Model file for the job. Use its own axes, mm. A direction names the side the tool comes from. Give positions to 0.01 mm unless a question says otherwise; leave off trailing zeros. Write each loop counter-clockwise with the first axis right and the second up, starting at its lowest first coordinate (ties: lowest second). Pieces come first, ordered by that corner, then holes. Notation, with made-up numbers: (60.5, -17.5) - (104.5, -17.5) arc R14 ccw to (104.5, -4.5) - close; hole circle Ø2 at (-20, 81.5). An arc over 180 degrees is marked (long way). One line per item, written item: value. Start each with the question number.
(1) Mould opens along Z. For faces 3 (the face through (-8.617, 13.461, 38.805)), 4 (the face through (-9.1, 28.575, -9.1)), 5 (the face through (-2.75, 22.31, 12.4)) say: pulls with the +Z half, pulls with the -Z half, needs draft (parallel to the pull), parting line crosses it, or undercut.
(2) Drop flat-ended pins along their axis: P1, Ø4.5, axis at x = 0, z = 51.63, coming from the +Y side; P2, Ø6, axis at x = 4.5, y = 20.5, coming from the -Z side; P3, Ø6, axis at x = -32.5, y = 9.5, coming from the +Z side. Give the stop position or say it passes through.
(3) Probe L1, parallel to Z at x = 0, y = -2; L2, parallel to X at y = 20.5, z = 0. List the from-to ranges inside material, lowest first.
(4) Cut at C-C, the plane y = 2. List the corners of the cut face in (x, z).
(5) Cut at A-A, the plane z = 0. List the corners of the cut face in (x, y) (3 decimals), and give its area (3 significant figures).
(6) Cut at B-B, the plane x = 0. List the corners of the cut face in (y, z) (3 decimals).
(7) 3-axis set-ups, long thin cutter, end or side, ignore diameter. For faces 1 (the face through (-38.4, 0, -11.7)), 2 (the face through (0.187, -4.829, -53.048)): which of +Z, -Z, +X, -X, +Y, -Y reach the whole face in a straight line?
(8) Cut at D-D, the plane y = 21.5. List the corners of the cut face in (x, z).
from build123d import *

# Parameters (mm, degrees)
SKETCH1_R                 = 39.749984
BOSS_EXTRUDE1_DEPTH       = 28.575
SKETCH3_R                 = 56.388
BOSS_EXTRUDE3_DEPTH       = 9.525
CHAMFER1_SIZE             = 1.27
TAP_DRILL_FOR_4_40_TAP1_D = 2.8702
SKETCH2_R                 = 12.7
CUT_EXTRUDE1_DEPTH        = 12.7


with BuildPart() as part:
    # Sketch1 → Boss-Extrude1 (new body)
    with BuildSketch(Plane(origin=(0, 0, 0), x_dir=(1, 0, 0), z_dir=(0, 1, 0))):
        Circle(SKETCH1_R)
    extrude(amount=BOSS_EXTRUDE1_DEPTH)

    # Sketch3 → Boss-Extrude3 (add)
    with BuildSketch(Plane.XZ):
        Circle(SKETCH3_R)
    extrude(amount=BOSS_EXTRUDE3_DEPTH)

    # Chamfer1
    chamfer1_edges = [part.edges().sort_by_distance(p)[0] for p in [
        (-39.749984, 28.575, 0),
    ]]
    chamfer(chamfer1_edges, length=CHAMFER1_SIZE)

    # Tap Drill for #4-40 Tap1 (through all)
    with Locations(Plane(origin=(0, 0, 0), x_dir=(1, 0, 0), z_dir=(0, 1, 0))):
        with Locations((0, 51.6255), (51.6255, 0), (0, -51.6255), (-51.6255, 0)):
            Hole(TAP_DRILL_FOR_4_40_TAP1_D / 2)

    # Sketch2 → Cut-Extrude1 (cut)
    with BuildSketch(Plane(origin=(0, 28.575, 0), x_dir=(1, 0, 0), z_dir=(0, 1, 0))):
        Circle(SKETCH2_R)
    extrude(amount=-CUT_EXTRUDE1_DEPTH, mode=Mode.SUBTRACT)


solid = part.part
Answers follow:
1. face 3: parting line crosses it
1. face 4: needs draft
1. face 5: undercut
2. P1: stops at y = 0
2. P2: stops at z = -39.72
2. P3: stops at z = 26.64
3. L1: z = -56.39 to -53.06, -50.19 to 50.19, 53.06 to 56.39
3. L2: x = -39.75 to -12.7, 12.7 to 39.75
4. outline: circle Ø79.5 at (0, 0)
5. outline: (-56.388, -9.525) - (-53.061, -9.525) - (-53.061, 0) - (-56.388, 0) - close; (-50.19, -9.525) - (50.19, -9.525) - (50.19, 0) - (39.75, 0) - (39.75, 27.305) - (38.48, 28.575) - (12.7, 28.575) - (12.7, 15.875) - (-12.7, 15.875) - (-12.7, 28.575) - (-38.48, 28.575) - (-39.75, 27.305) - (-39.75, 0) - (-50.19, 0) - close; (53.061, -9.525) - (56.388, -9.525) - (56.388, 0) - (53.061, 0) - close
5. area: 2,970 mm²
6. outline: (-9.525, -56.388) - (0, -56.388) - (0, -53.061) - (-9.525, -53.061) - close; (-9.525, -50.19) - (0, -50.19) - (0, -39.75) - (27.305, -39.75) - (28.575, -38.48) - (28.575, -12.7) - (15.875, -12.7) - (15.875, 12.7) - (28.575, 12.7) - (28.575, 38.48) - (27.305, 39.75) - (0, 39.75) - (0, 50.19) - (-9.525, 50.19) - close; (-9.525, 53.061) - (0, 53.061) - (0, 56.388) - (-9.525, 56.388) - close
7. face 1: +Y
7. face 2: +Y, -Y
8. outline: circle Ø79.5 at (0, 0); hole circle Ø25.4 at (0, 0)
